```python
from build123d import *

# Parameters (mm, degrees)
F0_W     = 47.423501
F0_H     = 18.892288
F2_DEPTH = 25


with BuildPart() as f1:
    # F0 (on Front) → F1 (revolve)
    with BuildSketch(Plane.XZ):
        with Locations((23.71175, 28.434824)):
            Rectangle(F0_W, F0_H)
    revolve(axis=Axis((23.71175, 0, 18.98868), (1, 0, 0)))

    # F0 (on Front) → F2 (join)
    with BuildSketch(Plane.XZ):
        Polygon((-74.412487, 54.845471), (-74.412487, 0), (0, 0), (0, 18.98868), (0, 37.880968), (0, 54.845471), align=None)
        with Locations((23.71175, 28.434824)):
            Rectangle(F0_W, F0_H)
    extrude(amount=F2_DEPTH)


solid = f1.part
```
The model under review builds one solid part; all positions refer to its coordinate system, in mm. A direction names the side the tool comes from. Round coordinates to 2 decimals unless told otherwise and drop trailing zeros. Write each loop counter-clockwise with the first axis right and the second up, starting at its lowest first coordinate (ties: lowest second). Pieces come first, ordered by that corner, then holes. Notation, with made-up numbers: (86, -4.75) - (114, -4.75) arc R28 ccw to (114, 14.25) - close; hole circle Ø2 at (-9.75, 6.5). An arc over 180 degrees is marked (long way). Use one line per item in the form item = value.
Q1. Consider section B-B (z = 17). State the section outline as (x, y) points, and give its area (3 significant figures).
Answer key:
outline = (-74.41, -25) - (0, -25) - (0, -18.79) - (47.42, -18.79) - (47.42, 18.79) - (0, 18.79) - (0, 0) - (-74.41, 0) - close
area = 3,640 mm2
Q2. Consider section C-C (x = 2). State the section outline as (y, z) points.
Answer key:
outline = (-25, 18.99) - (-18.89, 18.99) arc R18.89 ccw (long way) to (0, 37.88) - (-25, 37.88) - close
Q3. Consider section D-D (x = -25). State the section outline as (y, z) points.
Answer key:
outline = (-25, 0) - (0, 0) - (0, 54.85) - (-25, 54.85) - close
Q4. Consider section A-A (y = -21). State the section outline as (x, z) points.
Answer key:
outline = (-74.41, 0) - (0, 0) - (0, 18.99) - (47.42, 18.99) - (47.42, 37.88) - (0, 37.88) - (0, 54.85) - (-74.41, 54.85) - close
Q5. Insertion check: pin 1 Ø3 at (y, z) = (-17, 49) entering from +X; pin 2 Ø5 at (x, y) = (20.5, -22) entering from -Z; pin 3 Ø6 at (x, z) = (12.5, 39.5) entering from +Y. Each pin has a flat end and moves straight along its axis. Give the tip position at first contact, or say it passes through.
Answer key:
pin_1 = 0
pin_2 = 18.99
pin_3 = 7.09
Q6. Tool access review of faces 1 (the cylindrical face through (24.044, 12.911, 5.196)), 2 (the flat face through (0, -12, 46)), 3 (the flat face through (-38, 0, 28)), 4 (the flat face through (0, -18, 7)): name each direction out of +Z, -Z, +X, -X, +Y, -Y from which nothing blocks a thin tool from reaching the whole face with its end or side.
Answer key:
face_1 = +X
face_2 = +Z, +X, +Y, -Y
face_3 = +Z, -Z, -X, +Y
face_4 = -Z, +X, -Y
Q7. For line 1 (Y direction, x = -24.5, z = 25); line 2 (X direction, y = 6, z = 35.5); line 3 (X direction, y = -3, z = 45), list the stretches that pass through material, from the lowest coordinate up. Write a range as [from, to].
Answer key:
line_1 = [-25, 0]
line_2 = [0, 47.42]
line_3 = [-74.41, 0]
